```python
from build123d import *

# Parameters (mm, degrees)
CROQUIS1_R              = 2
SALIENTE_EXTRUIR1_DEPTH = 3.5
ROSCA1_PITCH            = 0.7
CROQUIS2_R              = 3.5
CROQUIS2_R_2            = 2.25
SALIENTE_EXTRUIR2_DEPTH = 2


with BuildPart() as part:
    # Croquis1 → Saliente-Extruir1 (new body)
    with BuildSketch(Plane(origin=(0, 0, 0), x_dir=(1, 0, 0), z_dir=(0, 1, 0))):
        Polygon((2.959554739, 4.957254188), (-2.81333069, 5.041676682), (-5.772885429, 0.084422494), (-2.959554739, -4.957254188), (2.81333069, -5.041676682), (5.772885429, -0.084422494), align=None)
        with Locations(Location((0, 0, 0), (0, 0, 270))):
            Circle(CROQUIS1_R, mode=Mode.SUBTRACT)
    extrude(amount=SALIENTE_EXTRUIR1_DEPTH)

    # Rosca1: the profile of Perfil de rosca1 profile screwed along a right-hand helix of 5 turns, 6 arcs to a turn; built about Z, then put on its axis
    rosca1_z = Axis((0, 0, 0), (0, 0, 1))
    rosca1_corners = [(1.9997, 0, -0.000173205), (2.378886113, 0, 0.218749999), (2.378886113, 0, 0.306249999), (1.9997, 0, 0.525173203)]
    with BuildLine(mode=Mode.PRIVATE) as rosca1_profile:
        Line(rosca1_corners[0], rosca1_corners[1])
        Line(rosca1_corners[1], rosca1_corners[2])
        Line(rosca1_corners[2], rosca1_corners[3])
        Line(rosca1_corners[3], rosca1_corners[0])
    rosca1_cap = Face(rosca1_profile.wire())
    rosca1_turn_angles = [0, 30, 60, 90, 120, 150, 180, 210, 240, 270, 300, 330, 360]
    rosca1_turn_weights = [1, 0.8660254037844387, 1, 0.8660254037844387, 1, 0.8660254037844387, 1, 0.8660254037844387, 1, 0.8660254037844387, 1, 0.8660254037844387, 1]
    rosca1_turn_rails = [Edge.make_bspline([Vector(p[0], p[1], 0).rotate(rosca1_z, rosca1_turn_angles[k]) / rosca1_turn_weights[k] + Vector(0, 0, p[2] + ROSCA1_PITCH * rosca1_turn_angles[k] / 360) for k in range(13)], [0, 0, 0, 1, 1, 2, 2, 3, 3, 4, 4, 5, 5, 6, 6, 6], 2, rosca1_turn_weights) for p in rosca1_corners]
    rosca1_turn_sides = [Face.make_surface_from_curves(rosca1_turn_rails[p[0]], rosca1_turn_rails[p[1]]) for p in [(0, 1), (1, 2), (2, 3), (3, 0)]]
    rosca1 = Plane(origin=(0, 3.5, 0), x_dir=(-1, 0, 0), z_dir=(0, -1, 0)) * Solid(Shell([*[p.moved(Location((0, 0, ROSCA1_PITCH * i))) for i in range(5) for p in rosca1_turn_sides], rosca1_cap, rosca1_cap.rotate(rosca1_z, 1800).moved(Location((0, 0, ROSCA1_PITCH * 1800 / 360)))]))
    add(rosca1, mode=Mode.SUBTRACT)

    # Croquis2 → Saliente-Extruir2 (add)
    with BuildSketch(Plane.XZ):
        with Locations(Location((0, 0, 0), (0, 0, 90))):
            Circle(CROQUIS2_R)
        with Locations(Location((0, 0, 0), (0, 0, 105.23750757))):
            Circle(CROQUIS2_R_2, mode=Mode.SUBTRACT)
    extrude(amount=SALIENTE_EXTRUIR2_DEPTH)


solid = part.part
```
The model under review builds one solid part; all positions refer to its coordinate system, in mm. A direction names the side the tool comes from. Round coordinates to 2 decimals unless told otherwise and drop trailing zeros. Loops run counter-clockwise (first coordinate to the right, second up) from the corner with the lowest first, then second, coordinate; pieces in that order, holes last. Notation, with made-up numbers: M 62.5,58.25 L 81.5,58.25 A10 cw 81.5,64.25 Z; hole C -4,-29.75 d1. An arc over 180 degrees is marked long. Write item = value, one per line.
Item 1: Take a section at D-D on x = 4.75. Write out the cut boundary in (y, z), then the cut area to 3 significant figures.
Return value:
outline = M 0,-1.75 L 3.5,-1.75 L 3.5,1.8 L 0,1.8 Z
area = 12.4 mm2
Item 2: Take a section at C-C on z = 4. Write out the cut boundary in (x, y).
Return value:
outline = M -3.49,0 L 3.44,0 L 3.44,3.5 L -3.49,3.5 Z
Item 3: Insertion check: P1, Ø1.5, axis at x = -1.5, y = -1, coming from the +Z side; P2, Ø3, axis at y = -1, z = 2.5, coming from the -X side. Each pin has a flat end and moves straight along its axis. Give the tip position at first contact, or say it passes through.
Return value:
P1 = 3.42
P2 = -4.95
Item 4: For line 1 (X direction, y = -1.25, z = 0); line 2 (Y direction, x = -1.5, z = -3.5); line 3 (Z direction, x = -1, y = -0.2), list the stretches that pass through material, from the lowest coordinate up. Write a range as [from, to].
Return value:
line_1 = [-3.5, -2.25], [2.25, 3.5]
line_2 = [0, 3.5]
line_3 = [-3.35, -2.02], [2.02, 3.35]
Item 5: Machinability: for faces 1 (the flat face through (4, 0, 0)), 2 (the flat face through (-4.27, 1.73, -2.6)), which of the approach directions +Z, -Z, +X, -X, +Y, -Y give a long, thin tool a straight path to every point of the face, cutting with its end or side? Answer none if there is none.
Return value:
face_1 = -Y
face_2 = -Z, -X, +Y, -Y
Item 6: The part is to be moulded in two halves that separate along X. For faces 3 (the flat face through (4.386, 1.726, -2.401)), 4 (the flat face through (-4.386, 1.726, 2.401)), 5 (the cylindrical face through (0.495, -0.986, -2.195)), 6 (the flat face through (2.5, 3.5, -0.1)), say which applies: released by +X, released by -X, zero draft, split by the parting line, or undercut.
Return value:
face_3 = released by +X
face_4 = released by -X
face_5 = undercut
face_6 = zero draft
Item 7: Take a section at A-A on y = -1.6. Write out the cut boundary in (x, z).
Return value:
outline = C 0,0 d7; hole C 0,0 d4.5
Item 8: Take a section at B-B on x = -3.25. Write out the cut boundary in (y, z).
Return value:
outline = M -2,-1.3 L 0,-1.3 L 0,-4.31 L 3.5,-4.31 L 3.5,4.44 L 0,4.44 L 0,1.3 L -2,1.3 Z
